Geometry check sheet. Reference: the model listing, model coordinates, mm. Give positions to 0.01 mm unless a question says otherwise; leave off trailing zeros. Order: outer loops, then holes, each group sorted by start corner. A loop starts at its lowest first (then second) coordinate and runs counter-clockwise, first axis right, second up. Notation, with made-up numbers: M 80.5,80.25 L 106.5,80.25 A29 cw 106.5,115.25 Z; hole C 20.25,-35 d8. An arc over 180 degrees is marked long. Answer as CSV lines item,"result". Start each with the question number.
```python
from build123d import *

# Parameters (mm, degrees)
SKETCH1_R           = 11.1
BUTTON_TOP_DEPTH    = 1.8
SKETCH2_R           = 11.1
SKETCH2_R_2         = 9.3
BUTTON_WALLS_DEPTH  = 4.8
STEM_HOUSING_DEPTH  = 4.6
CHAMFER1_SIZE       = 1.5
FILLET2_R           = 1
SKETCH8_R           = 13.2
SKETCH8_R_2         = 11.3
BOSS_EXTRUDE1_DEPTH = 2


with BuildPart() as part:
    # Sketch1 → button top (new body)
    with BuildSketch(Plane(origin=(0, 0, 0), x_dir=(1, 0, 0), z_dir=(0, 1, 0))):
        Circle(SKETCH1_R)
    extrude(amount=BUTTON_TOP_DEPTH)

    # Sketch2 → button walls (add)
    with BuildSketch(Plane(origin=(0, 1.8, 0), x_dir=(1, 0, 0), z_dir=(0, 1, 0))):
        Circle(SKETCH2_R)
        Circle(SKETCH2_R_2, mode=Mode.SUBTRACT)
    extrude(amount=BUTTON_WALLS_DEPTH)

    # Sketch3 → stem housing (add)
    with BuildSketch(Plane(origin=(0, 1.8, 0), x_dir=(1, 0, 0), z_dir=(0, 1, 0))):
        with BuildLine():
            ThreePointArc((3, 0), (2.597112711, -1.501667596), (1.496662955, -2.6))
            Line((1.496662955, -2.6), (3.6, -2.6))
            Line((3.6, -2.6), (3.6, 2.6))
            Line((3.6, 2.6), (1.496662955, 2.6))
            ThreePointArc((1.496662955, 2.6), (2.597112711, 1.501667596), (3, 0))
        make_face()
        with BuildLine():
            ThreePointArc((-1.496662955, 2.6), (-3, 0), (-1.496662955, -2.6))
            Line((-1.496662955, -2.6), (1.496662955, -2.6))
            ThreePointArc((1.496662955, -2.6), (2.597112711, -1.501667596), (3, 0))
            ThreePointArc((3, 0), (2.597112711, 1.501667596), (1.496662955, 2.6))
            Line((1.496662955, 2.6), (-1.496662955, 2.6))
        make_face()
        with BuildLine():
            ThreePointArc((-0.975, 0.675), (-0.762867966, 0.762867966), (-0.675, 0.975))
            Line((-0.675, 0.975), (-0.675, 2.1))
            Line((-0.675, 2.1), (0.675, 2.1))
            Line((0.675, 2.1), (0.675, 0.975))
            ThreePointArc((0.675, 0.975), (0.762867966, 0.762867966), (0.975, 0.675))
            Line((0.975, 0.675), (2.1, 0.675))
            Line((2.1, 0.675), (2.1, -0.675))
            Line((2.1, -0.675), (0.975, -0.675))
            ThreePointArc((0.975, -0.675), (0.762867966, -0.762867966), (0.675, -0.975))
            Line((0.675, -0.975), (0.675, -2.1))
            Line((0.675, -2.1), (-0.675, -2.1))
            Line((-0.675, -2.1), (-0.675, -0.975))
            ThreePointArc((-0.675, -0.975), (-0.762867966, -0.762867966), (-0.975, -0.675))
            Line((-0.975, -0.675), (-2.1, -0.675))
            Line((-2.1, -0.675), (-2.1, 0.675))
            Line((-2.1, 0.675), (-0.975, 0.675))
        make_face(mode=Mode.SUBTRACT)
        with BuildLine():
            Line((1.496662955, -2.6), (-1.496662955, -2.6))
            ThreePointArc((-1.496662955, -2.6), (0, -3), (1.496662955, -2.6))
        make_face()
        with BuildLine():
            Line((-3.6, 2.6), (-3.6, -2.6))
            Line((-3.6, -2.6), (-1.496662955, -2.6))
            ThreePointArc((-1.496662955, -2.6), (-3, 0), (-1.496662955, 2.6))
            Line((-1.496662955, 2.6), (-3.6, 2.6))
        make_face()
        with BuildLine():
            ThreePointArc((1.496662955, 2.6), (0, 3), (-1.496662955, 2.6))
            Line((-1.496662955, 2.6), (1.496662955, 2.6))
        make_face()
    extrude(amount=STEM_HOUSING_DEPTH)

    # Chamfer1
    chamfer1_edges = [part.edges().sort_by_distance(p)[0] for p in [
        (-9.3, 6.6, 0),
    ]]
    chamfer(chamfer1_edges, length=CHAMFER1_SIZE)

    # Fillet2
    fillet2_edges = [part.edges().sort_by_distance(p)[0] for p in [
        (3.6, 4.1, 2.6),
        (3.6, 4.1, -2.6),
        (-3.6, 4.1, -2.6),
        (-3.6, 4.1, 2.6),
    ]]
    fillet(fillet2_edges, radius=FILLET2_R)

    # Sketch6 → Cut-Revolve1 (revolve, cut)
    with BuildSketch(Plane.XY):
        with BuildLine():
            Line((-10.361522369, 0), (-10.561522369, 0.2))
            ThreePointArc((-10.561522369, 0.2), (-10.960054223, 0.79644507), (-11.1, 1.5))
            Line((-11.1, 1.5), (-11.1, 0))
            Line((-11.1, 0), (-10.361522369, 0))
        make_face()
    revolve(axis=Axis((0, 0, 0), (0, 1, 0)), mode=Mode.SUBTRACT)

    # Sketch7 → Revolve1 (revolve)
    with BuildSketch(Plane.XY):
        Polygon((11.1, 6.6), (12.7, 6.6), (11.1, 5), align=None)
    revolve(axis=Axis((0, 0, 0), (0, 1, 0)))

    # Sketch8 → Boss-Extrude1 (add)
    with BuildSketch(Plane(origin=(0, 6.6, 0), x_dir=(1, 0, 0), z_dir=(0, 1, 0))):
        Circle(SKETCH8_R)
        Circle(SKETCH8_R_2, mode=Mode.SUBTRACT)
    extrude(amount=BOSS_EXTRUDE1_DEPTH)


solid = part.part
```
Item 1: Section check A-A on y = 2.5. Give the number of separate pieces and of enclosed holes in the cut face, then the cut area to 3 significant figures.
Item 2: Section check D-D on y = 8. Record the boundary of the cut face in (x, z).
Item 3: Depth check by flat-ended pin: pin 1 Ø5 at (x, z) = (0.5, -1) entering from +Y; pin 2 Ø0.6 at (x, y) = (-2, 3.5) entering from -Z; pin 3 Ø4 at (x, y) = (-6.5, 6.5) entering from -Z. Enter the tip coordinate at first touch or a pass-through.
Item 4: Scan lines: line 1 along X through (y, z) = (2.5, 0); line 2 along Z through (x, y) = (0, 3.3); line 3 along X through (y, z) = (4.5, 0.75). Record each from-to range of solid material in increasing order.
Item 5: Draft check along X on faces 1 (the face through (0, 0, 0)), 2 (the face through (3.6, 4, 0)). Enter one of: pulls with the +X half, pulls with the -X half, needs draft (parallel to the pull), parting line crosses it, or undercut.
Numbers:
1,separate pieces,"2"
1,enclosed holes,"2"
1,area,"144 mm2"
2,outline,"C 0,0 d26.4; hole C 0,0 d22.6"
3,pin 1,"y = 6.4"
3,pin 2,"z = -10.97"
3,pin 3,"z = -12.41"
4,line 1,"-11.1 to -9.3, -3.6 to -2.1, 2.1 to 3.6, 9.3 to 11.1"
4,line 2,"-11.1 to -9.3, -3 to -2.1, 2.1 to 3, 9.3 to 11.1"
4,line 3,"-11.07 to -9.27, -3.6 to -0.78, 0.78 to 3.6, 9.27 to 11.07"
5,face 1,"needs draft"
5,face 2,"undercut"
